The figure shows three views and two pictorial views of one solid part (mm, origin at its lowest corner). Answer the questions. A direction names the side the tool comes from. Coordinates: 2 decimals unless noted, no trailing zeros. Loops run counter-clockwise (first coordinate to the right, second up) from the corner with the lowest first, then second, coordinate; pieces in that order, holes last. Notation, with made-up numbers: M -7,75.5 L 44,75.5 A25 cw 44,106.5 Z; hole C 54.5,-38.5 d1. An arc over 180 degrees is marked long. Answer as a JSON object with one key per item and string values. Group by question number.
1. A cutting plane is placed at A-A on y = 44.5. Give the vertices of the cut face in (x, z), and give its area (3 significant figures).
2. Given pin 1 (11 mm diameter, centred on x = 133.5, z = 46.5, fed in from -Y); pin 2 (4 mm diameter, centred on y = 25, z = 40, fed in from -X); pin 3 (5 mm diameter, centred on y = 56, z = 55.5, fed in from -X), each flat-ended and moving along its own axis, determine where each tip first touches the part or whether it passes through.
3. Straight lines are drawn through the part: L1, parallel to Y at x = 20, z = 5; L2, parallel to Z at x = 115, y = 57.6; L3, parallel to X at y = 56.45, z = 20. For each, find the intervals that lie inside material, in ascending order.
4. A cutting plane is placed at D-D on y = 30. Give the vertices of the cut face in (x, z).
5. A cutting plane is placed at B-B on x = 115. Give the vertices of the cut face in (y, z).
6. For the marked faces 4 and 5, determine the directions among +Z, -Z, +X, -X, +Y, -Y from which every point of the face is accessible in a straight line to the end or side of a thin tool.
7. Determine the mould class of the marked faces 1, 2 and 3 for opening direction Z: released by +Z, released by -Z, zero draft, split by the parting line, or undercut.
8. A cutting plane is placed at C-C on z = 20. Give the vertices of the cut face in (x, y).
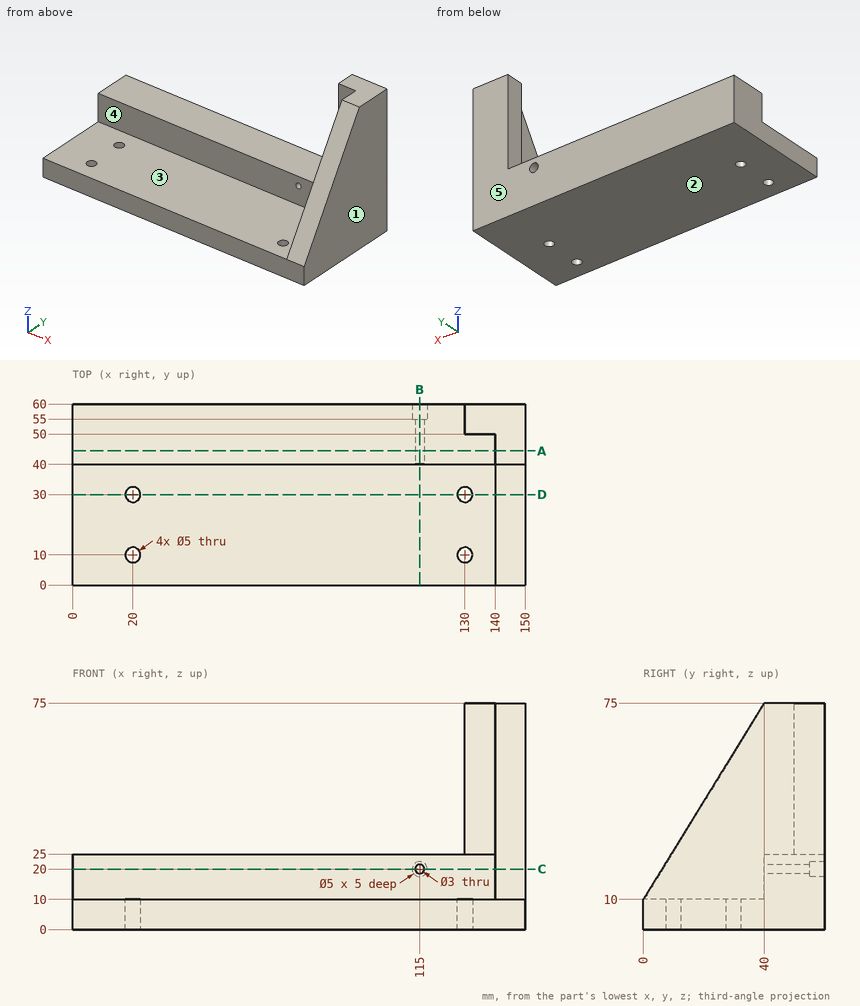
From the geometry:
{
 "1": {"outline": "M 0,0 L 150,0 L 150,75 L 140,75 L 140,25 L 0,25 Z; hole C 115,20 d3", "area": "4,240 mm²"},
 "2": {"pin 1": "stops at y = 50", "pin 2": "stops at x = 140", "pin 3": "stops at x = 130"},
 "3": {"L1": "y = 0 to 7.5, 12.5 to 27.5, 32.5 to 60", "L2": "z = 0 to 17.5, 22.5 to 25", "L3": "x = 0 to 112.5, 117.5 to 150"},
 "4": {"outline": "M 0,0 L 17.5,0 L 17.5,10 L 0,10 Z; M 22.5,0 L 127.5,0 L 127.5,10 L 22.5,10 Z; M 132.5,0 L 150,0 L 150,58.75 L 140,58.75 L 140,10 L 132.5,10 Z"},
 "5": {"outline": "M 0,0 L 60,0 L 60,17.5 L 55,17.5 L 55,18.5 L 40,18.5 L 40,10 L 0,10 Z; M 40,21.5 L 55,21.5 L 55,22.5 L 60,22.5 L 60,25 L 40,25 Z"},
 "6": {"face 4": "+Z, -X, -Y", "face 5": "+Z, -Z, +X, -X, +Y"},
 "7": {"face 1": "zero draft", "face 2": "released by -Z", "face 3": "released by +Z"},
 "8": {"outline": "M 0,40 L 113.5,40 L 113.5,55 L 112.5,55 L 112.5,60 L 0,60 Z; M 116.5,40 L 140,40 L 140,6.15 L 150,6.15 L 150,60 L 117.5,60 L 117.5,55 L 116.5,55 Z"}
}
